Build history of the part. All positions in model axes, mm. A direction names the side the tool comes from. Give positions to 0.01 mm unless a question says otherwise; leave off trailing zeros. Write each loop counter-clockwise with the first axis right and the second up, starting at its lowest first coordinate (ties: lowest second). Pieces come first, ordered by that corner, then holes. Notation, with made-up numbers: M -4,75.25 L 46,75.25 A8 ccw 46,79.25 Z; hole C 46,62.25 d7. An arc over 180 degrees is marked long. Return JSON: item names as keys, results as strings. Group by question number.
Q1. Flat gauge pins, fed straight in: pin 1 Ø5 at (x, z) = (-12.5, 15) entering from +Y; pin 2 Ø1.5 at (x, z) = (-5, -12) entering from -Y. Where does each tip first touch, or does it go through?
Q2. Band-saw the part on D-D, the plane x = -12.5. Give the cut face in (y, z).
Q3. Band-saw the part on B-B, the plane y = 2.8. Give the cut face in (x, z), then the cut area to 3 significant figures.
Q4. Pull direction Z, two halves, no side cores. Call faces 3 (the cylindrical face through (-11.277, 2.564, -12.649)), 4 (the flat face through (-25, 3, 0)), 5 (the cylindrical face through (24, 3, -23)), 6 (the cylindrical face through (13.723, 2.564, -12.649)): +Z half, -Z half, draft (parallel to the pull), parting line (faces both ways), or undercut.
Q5. Wall check: probe 1 along X at (y, z) = (3.7, 15); probe 2 along Z at (x, y) = (12.5, 1.3); probe 3 along Z at (x, y) = (6, 1.3). Give the ranges that are in metal, low to high.
Q6. Tool access for faces 1 (the flat face through (0, 3, -25)), 2 (the cylindrical face through (9.16, 2.56, 5.18)): list every direction of +Z, -Z, +X, -X, +Y, -Y with a clear straight run to the whole face (end or side of a thin tool).
Q7. Band-saw the part on C-C, the plane z = -15. Give the cut face in (x, y), then the cut area to 3 significant figures.
Q8. Band-saw the part on A-A, the plane x = 4. Give the cut face in (y, z).
from build123d import *

# Parameters (mm, degrees)
CROQUIS1_R              = 2.65
SALIENTE_EXTRUIR2_DEPTH = 8
CORTAR_EXTRUIR1_START   = 8
CROQUIS1_4_R            = 2.65
CORTAR_EXTRUIR1_DEPTH   = 2.8


with BuildPart() as part:
    # Croquis1 → Saliente-Extruir2 (new body)
    with BuildSketch(Plane(origin=(0, 0, 0), x_dir=(1, 0, 0), z_dir=(0, 1, 0))):
        with BuildLine():
            Line((-20, -25), (20, -25))
            ThreePointArc((20, -25), (23.535533906, -23.535533906), (25, -20))
            Line((25, -20), (25, 20))
            ThreePointArc((25, 20), (23.535533906, 23.535533906), (20, 25))
            Line((20, 25), (-20, 25))
            ThreePointArc((-20, 25), (-23.535533906, 23.535533906), (-25, 20))
            Line((-25, 20), (-25, -20))
            ThreePointArc((-25, -20), (-23.535533906, -23.535533906), (-20, -25))
        make_face()
        with Locations((-12.5, -15)):
            Circle(CROQUIS1_R, mode=Mode.SUBTRACT)
        with Locations((-12.5, 15)):
            Circle(CROQUIS1_R, mode=Mode.SUBTRACT)
        with Locations((12.5, -15)):
            Circle(CROQUIS1_R, mode=Mode.SUBTRACT)
        with Locations((12.5, 15)):
            Circle(CROQUIS1_R, mode=Mode.SUBTRACT)
        with BuildLine():
            Line((-7.060224725, -6.03567091), (7.060224725, -6.03567091))
            ThreePointArc((7.060224725, -6.03567091), (9.181545068, -5.156991253), (10.060224725, -3.03567091))
            Line((10.060224725, -3.03567091), (10.060224725, 3.03567091))
            ThreePointArc((10.060224725, 3.03567091), (9.181545068, 5.156991253), (7.060224725, 6.03567091))
            Line((7.060224725, 6.03567091), (-7.060224725, 6.03567091))
            ThreePointArc((-7.060224725, 6.03567091), (-9.181545068, 5.156991253), (-10.060224725, 3.03567091))
            Line((-10.060224725, 3.03567091), (-10.060224725, -3.03567091))
            ThreePointArc((-10.060224725, -3.03567091), (-9.181545068, -5.156991253), (-7.060224725, -6.03567091))
        make_face(mode=Mode.SUBTRACT)
    extrude(amount=SALIENTE_EXTRUIR2_DEPTH)

    # Croquis1<4> → Cortar-Extruir1 (cut)
    with BuildSketch(Plane(origin=(0, 0, 0), x_dir=(1, 0, 0), z_dir=(0, 1, 0)).offset(CORTAR_EXTRUIR1_START)):
        with BuildLine():
            Line((-20, -25), (20, -25))
            ThreePointArc((20, -25), (23.535533906, -23.535533906), (25, -20))
            Line((25, -20), (25, 20))
            ThreePointArc((25, 20), (23.535533906, 23.535533906), (20, 25))
            Line((20, 25), (-20, 25))
            ThreePointArc((-20, 25), (-23.535533906, 23.535533906), (-25, 20))
            Line((-25, 20), (-25, -20))
            ThreePointArc((-25, -20), (-23.535533906, -23.535533906), (-20, -25))
        make_face()
        with Locations((-12.5, -15)):
            Circle(CROQUIS1_4_R, mode=Mode.SUBTRACT)
        with Locations((-12.5, 15)):
            Circle(CROQUIS1_4_R, mode=Mode.SUBTRACT)
        with Locations((12.5, -15)):
            Circle(CROQUIS1_4_R, mode=Mode.SUBTRACT)
        with Locations((12.5, 15)):
            Circle(CROQUIS1_4_R, mode=Mode.SUBTRACT)
        with BuildLine():
            Line((-7.060224725, -6.03567091), (7.060224725, -6.03567091))
            ThreePointArc((7.060224725, -6.03567091), (9.181545068, -5.156991253), (10.060224725, -3.03567091))
            Line((10.060224725, -3.03567091), (10.060224725, 3.03567091))
            ThreePointArc((10.060224725, 3.03567091), (9.181545068, 5.156991253), (7.060224725, 6.03567091))
            Line((7.060224725, 6.03567091), (-7.060224725, 6.03567091))
            ThreePointArc((-7.060224725, 6.03567091), (-9.181545068, 5.156991253), (-10.060224725, 3.03567091))
            Line((-10.060224725, 3.03567091), (-10.060224725, -3.03567091))
            ThreePointArc((-10.060224725, -3.03567091), (-9.181545068, -5.156991253), (-7.060224725, -6.03567091))
        make_face(mode=Mode.SUBTRACT)
    extrude(amount=-CORTAR_EXTRUIR1_DEPTH, mode=Mode.SUBTRACT)


solid = part.part
From the geometry:
{
 "1": {"pin 1": "passes through", "pin 2": "stops at y = 0"},
 "2": {"outline": "M 0,-25 L 5.2,-25 L 5.2,-17.65 L 0,-17.65 Z; M 0,-12.35 L 5.2,-12.35 L 5.2,12.35 L 0,12.35 Z; M 0,17.65 L 5.2,17.65 L 5.2,25 L 0,25 Z"},
 "3": {"outline": "M -25,-20 A5 ccw -20,-25 L 20,-25 A5 ccw 25,-20 L 25,20 A5 ccw 20,25 L -20,25 A5 ccw -25,20 Z; hole C -12.5,-15 d5.3; hole C -12.5,15 d5.3; hole M -10.06,-3.04 A3 ccw -7.06,-6.04 L 7.06,-6.04 A3 ccw 10.06,-3.04 L 10.06,3.04 A3 ccw 7.06,6.04 L -7.06,6.04 A3 ccw -10.06,3.04 Z; hole C 12.5,-15 d5.3; hole C 12.5,15 d5.3", "area": "2,160 mm^2"},
 "4": {"face 3": "undercut", "face 4": "draft", "face 5": "-Z half", "face 6": "undercut"},
 "5": {"probe 1": "x = -25 to -15.15, -9.85 to 9.85, 15.15 to 25", "probe 2": "z = -25 to -17.65, -12.35 to 12.35, 17.65 to 25", "probe 3": "z = -25 to -6.04, 6.04 to 25"},
 "6": {"face 1": "-Z, +X, -X, +Y, -Y", "face 2": "+Y, -Y"},
 "7": {"outline": "M -25,0 L -15.15,0 L -15.15,5.2 L -25,5.2 Z; M -9.85,0 L 9.85,0 L 9.85,5.2 L -9.85,5.2 Z; M 15.15,0 L 25,0 L 25,5.2 L 15.15,5.2 Z", "area": "205 mm^2"},
 "8": {"outline": "M 0,-25 L 5.2,-25 L 5.2,-6.04 L 0,-6.04 Z; M 0,6.04 L 5.2,6.04 L 5.2,25 L 0,25 Z"}
}
